Geometry check sheet. Reference: the model listing, model coordinates, mm. A direction names the side the tool comes from. Round coordinates to 2 decimals unless told otherwise and drop trailing zeros. Order: outer loops, then holes, each group sorted by start corner. A loop starts at its lowest first (then second) coordinate and runs counter-clockwise, first axis right, second up.
(1) Gauge pin test, flat ends, axial feed: P1, Ø3, axis at x = 114.5, y = 85, coming from the +Z side; P2, Ø9.5, axis at x = 136.52, y = 74.63, coming from the -Z side; P3, Ø5, axis at x = 169.5, z = 2, coming from the +Y side; P4, Ø4, axis at x = 48, z = 23, coming from the -Y side. Record the tip position at first contact, or that the pin passes through.
(2) Cross-section at C-C on z = 63.5. Enter the section's corners in (x, y), and give its area (3 significant figures).
(3) Thickness scan on L1, parallel to Y at x = 64, z = 75; L2, parallel to X at y = 135, z = 73; L3, parallel to Z at x = 95.5, y = 32. Record the ranges inside material, lowest first.
(4) Cross-section at B-B on y = 107. Enter the section's corners in (x, z).
(5) Cross-section at A-A on x = 124.5. Enter the section's corners in (y, z), and give its area (3 significant figures).
(6) Draft check along X on faces 1 (the face through (86, 58, 6.35)), 2 (the face through (68.26, 76.6, 3.13)), 3 (the face through (159.004, 169, 75)), 4 (the face through (141.676, 74.398, 3.131)). Enter one of: pulls with the +X half, pulls with the -X half, needs draft (parallel to the pull), parting line crosses it, or undercut.
(7) Set-up check for faces 5 (the face through (103, 114.3, 78)), 6 (the face through (167, 114.3, 3)), 7 (the face through (24, 114.3, 3)): record each of +Z, -Z, +X, -X, +Y, -Y from which the full face is reachable in a straight line by a thin tool's end or side.
from build123d import *

# Parameters (mm, degrees)
SKETCH1_W           = 174.752
SKETCH1_H           = 114.3
BOSS_EXTRUDE1_DEPTH = 6.35
SKETCH2_W           = 111.252
SKETCH2_H           = 111.252
BOSS_EXTRUDE2_DEPTH = 152.4
SKETCH3_R           = 5.1562
CUT_EXTRUDE1_DEPTH  = 324.47755132


with BuildPart() as part:
    # Sketch1 → Boss-Extrude1 (new body)
    with BuildSketch(Plane.XY):
        with Locations((87.376, 57.15)):
            Rectangle(SKETCH1_W, SKETCH1_H)
    extrude(amount=BOSS_EXTRUDE1_DEPTH)

    # Sketch2 → Boss-Extrude2 (add)
    with BuildSketch(Plane.XY):
        with Locations((103.378, 169.926)):
            Rectangle(SKETCH2_W, SKETCH2_H)
    extrude(amount=BOSS_EXTRUDE2_DEPTH)

    # Sketch3 → Cut-Extrude1 (cut, through all)
    with BuildSketch(Plane.XY):
        with Locations(Location((73.025, 74.6252, 0), (0, 0, 180))):
            Circle(SKETCH3_R)
        with Locations(Location((136.525, 74.6252, 0), (0, 0, 180))):
            Circle(SKETCH3_R)
    extrude(amount=CUT_EXTRUDE1_DEPTH, mode=Mode.SUBTRACT)


solid = part.part
Found:
1. P1: stops at z = 6.35
1. P2: passes through
1. P3: stops at y = 114.3
1. P4: stops at y = 114.3
2. outline: (47.75, 114.3) - (159, 114.3) - (159, 225.55) - (47.75, 225.55) - close
2. area: 12,400 mm2
3. L1: y = 114.3 to 225.55
3. L2: x = 47.75 to 159
3. L3: z = 0 to 6.35
4. outline: (0, 0) - (174.75, 0) - (174.75, 6.35) - (0, 6.35) - close
5. outline: (0, 0) - (225.55, 0) - (225.55, 152.4) - (114.3, 152.4) - (114.3, 6.35) - (0, 6.35) - close
5. area: 17,700 mm2
6. face 1: needs draft
6. face 2: undercut
6. face 3: pulls with the +X half
6. face 4: undercut
7. face 5: +Z, +X, -X, -Y
7. face 6: +Z, -Z, +X, +Y
7. face 7: +Z, -Z, -X, +Y
